from build123d import *

# Parameters (mm, degrees)
F0_R     = 35
F1_DEPTH = 100
F2_T     = -2
F5_R     = 10


# Not quite as in the source:
# - a fillet or chamfer that OpenCascade refuses, or shapes differently, is made with other operations: its cross-section is extruded or revolved along the edge and cut away or added


with BuildPart() as f1:
    # F0 (on Top) → F1 (new body)
    with BuildSketch(Plane.XY):
        Circle(F0_R)
    extrude(amount=F1_DEPTH)

    # F2
    f2_openings = [f1.faces().sort_by_distance(p)[0] for p in [
        (0, 0, 100),
    ]]
    offset(amount=F2_T, openings=f2_openings)

    # F3: fillet of radius 5 on 1 edges, made by hand

    # F3_s1 → F3_t2 (revolve, cut)
    with BuildSketch(Plane.XZ):
        with BuildLine():
            ThreePointArc((35, 96), (34.472135955, 98.2360679775), (33, 100))
            Line((33, 100), (35, 100))
            Line((35, 100), (35, 96))
        make_face()
    revolve(axis=Axis((0, 0, 100), (0, 0, 1)), mode=Mode.SUBTRACT)

    # F4: fillet of radius 1 on 1 edges, made by hand

    # F4_s1 → F4_t2 (revolve, cut)
    with BuildSketch(Plane.XZ):
        with BuildLine():
            ThreePointArc((35, 96.0000100581), (33.9999989942, 97.0000080465), (33, 96.0000080465))
            Line((33, 96.0000080465), (33, 100))
            ThreePointArc((33, 100), (34.4721337059, 98.2360724756), (35, 96.0000100581))
        make_face()
    revolve(axis=Axis((0, 0, 100), (0, 0, 1)), mode=Mode.SUBTRACT)

    # F5
    f5_edges = [f1.edges().sort_by_distance(p)[0] for p in [
        (-33, 0, 2),
    ]]
    fillet(f5_edges, radius=F5_R)


solid = f1.part
Design review of the part built by this model. Coordinates are the model's own, in mm. Round coordinates to 2 decimals unless told otherwise and drop trailing zeros. Write each loop counter-clockwise with the first axis right and the second up, starting at its lowest first coordinate (ties: lowest second). Pieces come first, ordered by that corner, then holes.
Item 1: Wall thickness on L1, parallel to Y at x = 0, z = 55; L2, parallel to Z at x = 2, y = 19; L3, parallel to Y at x = -22.5, z = 92.5: over which ranges is each line inside the solid? List them lowest first.
Item 2: For pin 1 Ø4 at (y, z) = (10.5, 53.5) entering from +X; pin 2 Ø8 at (y, z) = (-26.5, 28) entering from +X; pin 3 Ø1.5 at (x, y) = (-4, -27) entering from +Z, all flat-tipped, find the tip position at first contact; note any pin that passes through.
Item 3: Consider section D-D on z = 10. Give the boundary of the cut face in (x, y), and give its area (3 significant figures).
Item 4: Consider section B-B on z = 56. Give the boundary of the cut face in (x, y).
Item 5: Draft analysis for pull direction Y (two halves, no side actions). For faces 1 (the flat face through (0, 0, 0)), 2 (the cylindrical face through (30.5, -12.6, 53.4)), 3 (the cylindrical face through (-28, -21, 47)), state which applies: released by +Y, released by -Y, zero draft, split by the parting line, or undercut.
Check values:
1. L1: y = -35 to -33, 33 to 35
1. L2: z = 0 to 2
1. L3: y = -26.81 to -24.14, 24.14 to 26.81
2. pin 1: stops at x = 33.95
2. pin 2: stops at x = 26.81
2. pin 3: stops at z = 3.37
3. outline: circle Ø70 at (0, 0); hole circle Ø65.6 at (0, 0)
3. area: 469 mm2
4. outline: circle Ø70 at (0, 0); hole circle Ø66 at (0, 0)
5. face 1: zero draft
5. face 2: undercut
5. face 3: split by the parting line
